For this review, use the dimensioned drawing (mm, ordinates from the lowest corner) and the shaded views. A direction names the side the tool comes from. Round coordinates to 2 decimals unless told otherwise and drop trailing zeros. Write each loop counter-clockwise with the first axis right and the second up, starting at its lowest first coordinate (ties: lowest second). Pieces come first, ordered by that corner, then holes. Notation, with made-up numbers: (61.5, 64.5) - (79.5, 64.5) arc R23 cw to (79.5, 74.5) - close; hole circle Ø11 at (22, 46). An arc over 180 degrees is marked (long way). Write each question's results on one line, items separated by ' | '.
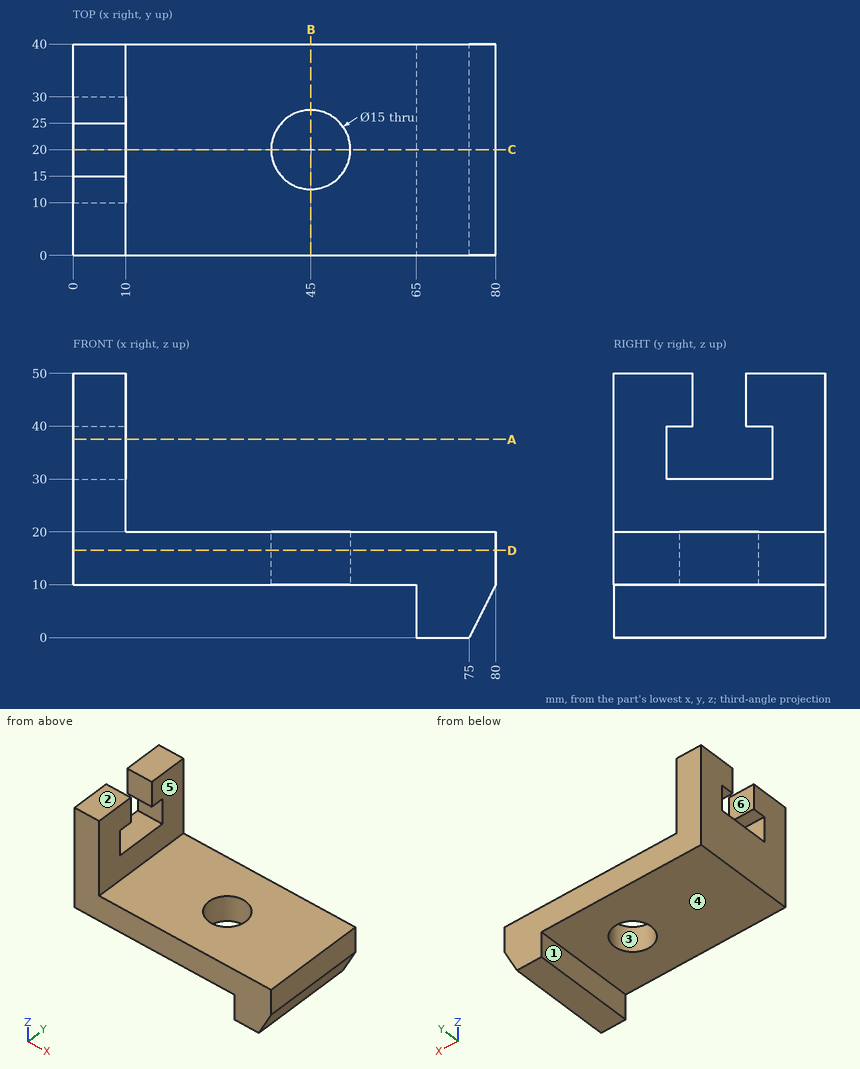
Q1. The part is to be moulded in two halves that separate along X. For the marked faces 1, 2 and 3, say which applies: released by +X, released by -X, zero draft, split by the parting line, or undercut.
Evaluation:
face 1: released by -X | face 2: zero draft | face 3: undercut
Q2. We need section B-B (x = 45). State the section outline as (y, z) points.
Evaluation:
outline: (0, 10) - (12.5, 10) - (12.5, 20) - (0, 20) - close; (27.5, 10) - (40, 10) - (40, 20) - (27.5, 20) - close
Q3. Insertion check: P1, Ø3, axis at x = 63, y = 25, coming from the +Z side; P2, Ø3, axis at x = 3.5, y = 20, coming from the +Z side; P3, Ø5.5, axis at x = 5, y = 13, coming from the -Z side; P4, Ø9, axis at x = 45, y = 20, coming from the +Z side. Each pin has a flat end and moves straight along its axis. Give the tip position at first contact, or say it passes through.
Evaluation:
P1: stops at z = 20 | P2: stops at z = 30 | P3: stops at z = 10 | P4: passes through
Q4. For probe 1 along Y at (x, z) = (45, 18); probe 2 along Z at (x, y) = (8, 12.5); probe 3 along Z at (x, y) = (47, 35), list the stretches that pass through material, from the lowest coordinate up.
Evaluation:
probe 1: y = 0 to 12.5, 27.5 to 40 | probe 2: z = 10 to 30, 40 to 50 | probe 3: z = 10 to 20
Q5. Tool access review of the marked faces 4, 5 and 6: name each direction out of +Z, -Z, +X, -X, +Y, -Y from which nothing blocks a thin tool from reaching the whole face with its end or side.
Evaluation:
face 4: -Z, -X, +Y, -Y | face 5: +Z, +X, +Y, -Y | face 6: +Z, +X, -X
Q6. We need section A-A (z = 37.5). State the section outline as (x, y) points, plus the area to 3 significant figures.
Evaluation:
outline: (0, 0) - (10, 0) - (10, 10) - (0, 10) - close; (0, 30) - (10, 30) - (10, 40) - (0, 40) - close | area: 200 mm^2
Q7. We need section C-C (y = 20). State the section outline as (x, z) points, plus the area to 3 significant figures.
Evaluation:
outline: (0, 10) - (37.5, 10) - (37.5, 20) - (10, 20) - (10, 30) - (0, 30) - close; (52.5, 10) - (65, 10) - (65, 0) - (75, 0) - (80, 10) - (80, 20) - (52.5, 20) - close | area: 875 mm^2
Q8. We need section D-D (z = 16.5). State the section outline as (x, y) points.
Evaluation:
outline: (0, 0) - (80, 0) - (80, 40) - (0, 40) - close; hole circle Ø15 at (45, 20)
